Autodesk Inventor part; units mm, degrees
ref_plane "YZ Plane" through (0, 0, 0) normal (1, 0, 0) x (0, 1, 0)
ref_plane "XZ Plane" through (0, 0, 0) normal (0, 1, 0) x (-1, 0, 0)
ref_plane "XY Plane" through (0, 0, 0) normal (0, 0, 1) x (1, 0, 0)
sketch "Эскиз" plane through (0, 0, 0) normal (1, 0, 0) x (0, 1, 0)
  circle A0 centre (0, 0) radius 3
  dimension "d1" = 6
extrude "Базовый элемент" add sketch "Эскиз" along normal blind 40
chamfer "Фаска1" distance 2 angle 30 1 edges at (0, -3, 0) measured on face at (26.6667, 2.9612, -0.4812)
chamfer "Эскиз2" distance 2 angle 30 1 edges at (40, -3, 0) measured on face at (27.3333, 2.9903, -0.2414)
sketch "Эскиз3" plane through (0, 0, 0) normal (0, 1, 0) x (-1, 0, 0)
  line L0 (0, 1.8453) -> (0, -1.8453) construction
  line L1 (-40, -1.8453) -> (-40, 1.8453) construction
  line L2 (-2, -3) -> (-38, -3) construction
  line L3 (8, 0) -> (-48, 0) construction
  line L4 (0, -4.2) -> (0, 4.2) construction
  line L5 (-7.5, 9) -> (-32.5, 9) construction
  line L6 (-32.5, 9) -> (-32.5, -9) construction
  line L7 (-32.5, -9) -> (-7.5, -9) construction
  line L8 (-7.5, -9) -> (-7.5, 9) construction
  line L9 (-7.5, -2.7) -> (-8.3, -2.7)
  line L10 (-8.3, -2.7) -> (-8.3, -7)
  line L11 (-8.3, -7) -> (-7.5, -7)
  line L12 (-7.5, -7) -> (-7.5, -2.7)
  point P0 (0, 0)
  dimension "d17" = 25
  dimension "d18" = 7.5
  dimension "d19" = 18
  dimension "d20" = 9
  dimension "d21" = 0.8
  dimension "d22" = 2.7
  dimension "d23" = 7
revolve "Вращение1" cut sketch "Эскиз3" angle 360 about axis through (-10, 0, 0) along (1, 0, 0)
equation "\"d1\" = NND"
equation "\"d2\" = NLG"
equation "\"d8\" = PHH"
equation "\"d9\" = FAWI"
equation "\"d12\" = PHH"
equation "\"d4\" = PHH"
equation "\"d5\" = FAWI"
equation "\"d11\" = PHH"
equation "\"NND\" = 6"
equation "\"NLG\" = 40"
equation "\"PHH\" = 2"
equation "\"FAWI\" = 30deg"
equation "\"DIST1\" = 3.2"
equation "\"DIST2\" = DIST1"
equation "\"BOR1\" = 1.6"
equation "\"FAWI2\" = 30deg"
equation "\"BOR2\" = BOR1"
equation "\"PHH2\" = PHH"
properties part number "ISO 2340 - A - 6 x 40" material "Сталь"
Here's how the part is built. I have some questions about the finished solid (model axes, mm). Give positions to 0.01 mm unless a question says otherwise; leave off trailing zeros. Write each loop counter-clockwise with the first axis right and the second up, starting at its lowest first coordinate (ties: lowest second). Pieces come first, ordered by that corner, then holes. Notation, with made-up numbers: M 32,78.5 L 80,78.5 A19 ccw 80,90.5 Z; hole C 38,76.25 d9. An arc over 180 degrees is marked long. Put each result on its own line as item: value. Start each with the question number.
Item 1: Thinking about a two-plate mould opening in X: for faces 1 (the cylindrical face through (7.906, -2.636, 0.585)), 2 (the conical face through (0.13, -1.92, 0.08)), 3 (the cylindrical face through (5, -3, 0)), 4 (the flat face through (40, 0, 0)), which applies, +X half, -X half, draft (parallel to the pull), parting line (faces both ways), or undercut?
Item 2: Will this pin go through, and if not, where does the flat tip stop? pin 1 (2 mm diameter, centred on x = 20, z = -2, fed in from +Y).
Item 3: If we section it at C-C, the plane x = 4: Write out the boundary of the cut face in (y, z), then the cut area to 3 significant figures.
Item 4: I need wall thicknesses on L1, parallel to Y at x = 2.5, z = 0.1; L2, parallel to Z at x = 16, y = 0.2; L3, parallel to X at y = -2.1, z = -1.75. Which ranges of each line are inside material? Lowest first, please. Write a range as from..to.
Item 5: If we section it at A-A, the plane z = 0: Write out the boundary of the cut face in (x, y), then the cut area to 3 significant figures.
Values:
1. face 1: undercut
1. face 2: -X half
1. face 3: draft
1. face 4: +X half
2. pin 1: y = 2.83
3. outline: C 0,0 d6
3. area: 28.3 mm²
4. L1: -3..3
4. L2: -2.99..2.99
4. L3: 1.54..7.5, 8.3..38.46
5. outline: M 0,-1.85 L 2,-3 L 7.5,-3 L 7.5,-2.7 L 8.3,-2.7 L 8.3,-3 L 38,-3 L 40,-1.85 L 40,1.85 L 38,3 L 8.3,3 L 8.3,2.7 L 7.5,2.7 L 7.5,3 L 2,3 L 0,1.85 Z
5. area: 235 mm²
